Print and shaded views of the part. All mm, measured from the part's lowest x, y and z. Give positions to 0.01 mm unless a question says otherwise; leave off trailing zeros. Loops run counter-clockwise (first coordinate to the right, second up) from the corner with the lowest first, then second, coordinate; pieces in that order, holes last. Notation, with made-up numbers: (-37.75, -9) - (-10.75, -9) arc R22 ccw to (-10.75, 20) - close; hole circle Ø5 at (-16, 77.25). An arc over 180 degrees is marked (long way). Return JSON: item names as keys, results as strings.
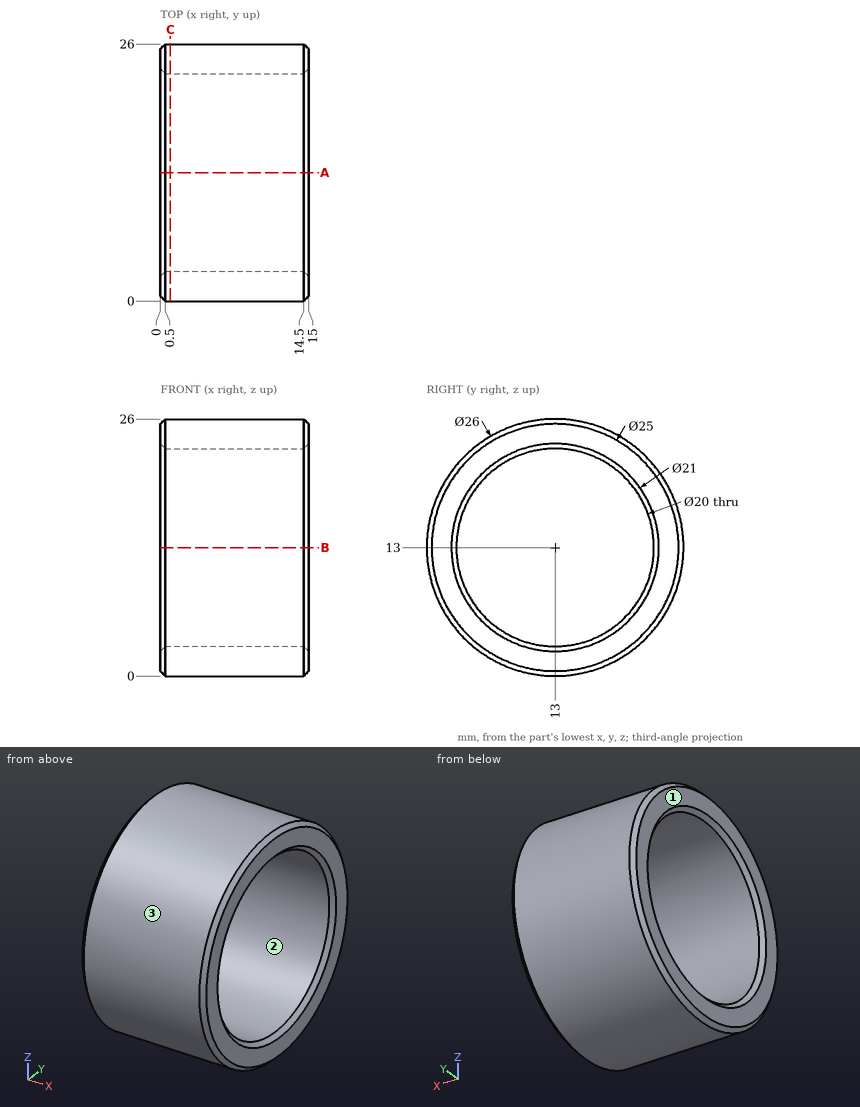
1. Pull direction Y, two halves, no side cores. Call the marked faces 1, 2 and 3: +Y half, -Y half, draft (parallel to the pull), parting line (faces both ways), or undercut.
Values follow:
{"face 1": "draft", "face 2": "undercut", "face 3": "parting line"}
2. Drop flat-ended pins along their axis: P1, Ø2, axis at x = 7, y = 5, coming from the +Z side; P2, Ø8, axis at x = 7.5, y = 13.5, coming from the -Z side; P3, Ø1, axis at x = 9, z = 8, coming from the -Y side; P4, Ø3, axis at x = 11, z = 21.5, coming from the +Y side. Give the stop position or say it passes through.
Values follow:
{"P1": "stops at z = 23.95", "P2": "stops at z = 0", "P3": "stops at y = 0.8", "P4": "stops at y = 23.95"}
3. Cut at C-C, the plane x = 1. Write the cut outline in (y, z), plus the area to 3 significant figures.
Values follow:
{"outline": "circle Ø26 at (13, 13); hole circle Ø20 at (13, 13)", "area": "217 mm²"}
4. Cut at A-A, the plane y = 13. Write the cut outline in (x, z).
Values follow:
{"outline": "(0, 0.5) - (0.5, 0) - (14.5, 0) - (15, 0.5) - (15, 2.5) - (14.5, 3) - (0.5, 3) - (0, 2.5) - close; (0, 23.5) - (0.5, 23) - (14.5, 23) - (15, 23.5) - (15, 25.5) - (14.5, 26) - (0.5, 26) - (0, 25.5) - close"}
5. Drill centre lines: probe 1 along Y at (x, z) = (7.75, 13); probe 2 along Z at (x, y) = (11, 7); probe 3 along Y at (x, z) = (12.5, 17.5). Where is each one in solid material? Low to high.
Values follow:
{"probe 1": "y = 0 to 3, 23 to 26", "probe 2": "z = 1.47 to 5, 21 to 24.53", "probe 3": "y = 0.8 to 4.07, 21.93 to 25.2"}
